```python
from build123d import *

# Parameters (mm, degrees)
SKETCH_1_R      = 4.1
EXTRUDE_1_DEPTH = 21.5
FILLET_1_R      = 15


with BuildPart() as part:
    # Sketch 1 → Extrude 1 (new, symmetric)
    with BuildSketch(Plane.XY):
        with BuildLine():
            Line((-220.71165321, 37.734887356), (-60.125305402, 52.28709885))
            ThreePointArc((-60.125305402, 52.28709885), (-79.680568873, 0), (-60.125305402, -52.28709885))
            Line((-60.125305402, -52.28709885), (-220.71165321, -37.734887356))
            ThreePointArc((-220.71165321, -37.734887356), (-204.013605252, 0), (-220.71165321, 37.734887356))
        make_face()
        with Locations((-192.444390405, 21)):
            Circle(SKETCH_1_R, mode=Mode.SUBTRACT)
        with Locations((-192.444390405, -21)):
            Circle(SKETCH_1_R, mode=Mode.SUBTRACT)
        with Locations((-92.32231649, -21)):
            Circle(SKETCH_1_R, mode=Mode.SUBTRACT)
        with Locations((-92.32231649, 21)):
            Circle(SKETCH_1_R, mode=Mode.SUBTRACT)
    extrude(amount=EXTRUDE_1_DEPTH, both=True)

    # Fillet 1
    fillet_1_edges = [part.edges().sort_by_distance(p)[0] for p in [
        (-220.71165321, 37.734887356, 0),
        (-60.125305402, 52.28709885, 0),
        (-60.125305402, -52.28709885, 0),
        (-220.71165321, -37.734887356, 0),
    ]]
    fillet(fillet_1_edges, radius=FILLET_1_R)


solid = part.part
```
Geometry: final body of the model. Coordinates: model frame, mm. Coordinates: 2 decimals unless noted, no trailing zeros. Write each loop counter-clockwise with the first axis right and the second up, starting at its lowest first coordinate (ties: lowest second). Pieces come first, ordered by that corner, then holes. Notation, with made-up numbers: M 88,-20 L 116,-20 A13 ccw 116,5 Z; hole C 55,52 d3. An arc over 180 degrees is marked long. Answer as CSV lines item,"result". Start each with the question number.
Q1. Cut plane D-D on y = -37. Return the cut outline in (x, z), then the cut area to 3 significant figures.
Q2. Pin query (flat end, axial travel): P1, Ø7.5, axis at x = -192.44, y = -21, coming from the -Z side; P2, Ø6, axis at x = -99, z = -7.5, coming from the +Y side; P3, Ø5, axis at y = 22, z = 2, coming from the +X side; P4, Ø6, axis at x = -117, z = 2, coming from the -Y side (3 decimals). Return the tip coordinate at first contact, or that it passes through.
Q3. Cut plane C-C on x = -182.5. Return the cut outline in (y, z).
Q4. Cut plane B-B on y = 21. Return the cut outline in (x, z), then the cut area to 3 significant figures.
Q5. Cut plane A-A on z = 18. Return the cut outline in (x, y), then the cut area to 3 significant figures.
Q6. Line query: line 1 (Y direction, x = -192, z = -3); line 2 (Y direction, x = -89, z = 8); line 3 (X direction, y = -29, z = 3). Output: solid intervals per line, ascending. Write a range as from..to.
Q7. Mould query, pull axis X, two halves, no side actions, for faces 1 (the cylindrical face through (-196.54, -20.82, -0.3)), 2 (the cylindrical face through (-79.68, 0.42, 0.3)), 3 (the flat face through (-140, 1, 21.5)), 4 (the flat face through (-143.129, 44.765, 0.301)). Classes: released by +X, released by -X, zero draft, split by the parting line, or undercut.
Findings below:
1,outline,"M -203.1,-21.5 L -73.28,-21.5 L -73.28,21.5 L -203.1,21.5 Z"
1,area,"5,580 mm2"
2,P1,"passes through"
2,P2,"stops at y = 49.04"
2,P3,"stops at x = -75.82"
2,P4,"stops at y = -47.405"
3,outline,"M -41.2,-21.5 L 41.2,-21.5 L 41.2,21.5 L -41.2,21.5 Z"
4,outline,"M -208.4,-21.5 L -196.54,-21.5 L -196.54,21.5 L -208.4,21.5 Z; M -188.34,-21.5 L -96.42,-21.5 L -96.42,21.5 L -188.34,21.5 Z; M -88.22,-21.5 L -76.86,-21.5 L -76.86,21.5 L -88.22,21.5 Z"
4,area,"4,950 mm2"
5,outline,"M -207.85,-19.39 A15 ccw -195.33,-40.04 L -89.45,-49.63 A15 ccw -74.14,-29.19 A79.68 cw -74.14,29.19 A15 ccw -89.45,49.63 L -195.33,40.04 A15 ccw -207.85,19.39 A50.99 cw Z; hole C -192.44,-21 d8.2; hole C -192.44,21 d8.2; hole C -92.32,-21 d8.2; hole C -92.32,21 d8.2"
5,area,"11,400 mm2"
6,line 1,"y = -40.34..-25.08, -16.92..16.92, 25.08..40.34"
6,line 2,"y = -49.66..-23.4, -18.6..18.6, 23.4..49.66"
6,line 3,"x = -208.46..-74.22"
7,face 1,"undercut"
7,face 2,"released by +X"
7,face 3,"zero draft"
7,face 4,"released by -X"
